from build123d import *

# Parameters (mm, degrees)
SKETCH_1_W          = 15.8
SKETCH_1_H          = 7.8
SKETCH_1_R          = 2.4
EXTRUDE_1_DEPTH     = 3.2
SKETCH_2_R          = 2.4
SKETCH_2_R_2        = 1.6
EXTRUDE_2_DEPTH     = 1.7
SKETCH_3_R          = 2.5
CUT_EXTRUDE_2_DEPTH = 1.8


with BuildPart() as part:
    # Эскиз1 → Бобышка-Вытянуть1 (new body)
    # profile 1 of 2: a face of its own
    with BuildSketch(Plane(origin=(0, 0, 0), x_dir=(1, 0, 0), z_dir=(0, 1, 0))):
        Rectangle(SKETCH_1_W, SKETCH_1_H)
        Circle(SKETCH_1_R, mode=Mode.SUBTRACT)
    # profile 2 of 2: a face of its own
    with BuildSketch(Plane(origin=(0, 0, 0), x_dir=(1, 0, 0), z_dir=(0, 1, 0))):
        Circle(SKETCH_1_R)
    extrude(amount=EXTRUDE_1_DEPTH)

    # Эскиз2 → Бобышка-Вытянуть2 (add)
    with BuildSketch(Plane(origin=(0, 0, 0), x_dir=(1, 0, 0), z_dir=(0, 1, 0))):
        with Locations(Location((0, 0, 0), (0, 0, 270))):
            Circle(SKETCH_2_R)
        with Locations(Location((0, 0, 0), (0, 0, 270))):
            Circle(SKETCH_2_R_2, mode=Mode.SUBTRACT)
    extrude(amount=-EXTRUDE_2_DEPTH)

    # Эскиз3 → Вырез-Вытянуть2 (cut)
    with BuildSketch(Plane(origin=(0, 3.2, 0), x_dir=(1, 0, 0), z_dir=(0, 1, 0))):
        with Locations(Location((-4, 0, 0), (0, 0, 270))):
            Circle(SKETCH_3_R)
        with Locations(Location((4, 0, 0), (0, 0, 270))):
            Circle(SKETCH_3_R)
    extrude(amount=-CUT_EXTRUDE_2_DEPTH, mode=Mode.SUBTRACT)


solid = part.part
The model under review builds one solid part; all positions refer to its coordinate system, in mm. A direction names the side the tool comes from. Round coordinates to 2 decimals unless told otherwise and drop trailing zeros. Order: outer loops, then holes, each group sorted by start corner. A loop starts at its lowest first (then second) coordinate and runs counter-clockwise, first axis right, second up. Notation, with made-up numbers: (-32, 41.25) -> (5, 41.25) arc R15 cw to (5, 62.25) -> close; hole circle Ø1 at (-21, 46). An arc over 180 degrees is marked (long way). Return JSON: item names as keys, results as strings.
1. For L1, parallel to X at y = 2.7, z = 0; L2, parallel to X at y = -0.35, z = 0; L3, parallel to X at y = 2.4, z = -0.75, list the stretches that pass through material, from the lowest coordinate up. Write a range as [from, to].
Answer block:
{"L1": "x = [-7.9, -6.5], [-1.5, 1.5], [6.5, 7.9]", "L2": "x = [-2.4, -1.6], [1.6, 2.4]", "L3": "x = [-7.9, -6.38], [-1.62, 1.62], [6.38, 7.9]"}
2. Take a section at C-C (y = 2.85). Write out the cut boundary in (x, z).
Answer block:
{"outline": "(-7.9, -3.9) -> (7.9, -3.9) -> (7.9, 3.9) -> (-7.9, 3.9) -> close; hole circle Ø5 at (-4, 0); hole circle Ø5 at (4, 0)"}
3. Take a section at A-A (z = 0). Write out the cut boundary in (x, y), then the cut area to 3 significant figures.
Answer block:
{"outline": "(-7.9, 0) -> (-2.4, 0) -> (-2.4, -1.7) -> (-1.6, -1.7) -> (-1.6, 0) -> (1.6, 0) -> (1.6, -1.7) -> (2.4, -1.7) -> (2.4, 0) -> (7.9, 0) -> (7.9, 3.2) -> (6.5, 3.2) -> (6.5, 1.4) -> (1.5, 1.4) -> (1.5, 3.2) -> (-1.5, 3.2) -> (-1.5, 1.4) -> (-6.5, 1.4) -> (-6.5, 3.2) -> (-7.9, 3.2) -> close", "area": "35.3 mm²"}
4. Take a section at D-D (y = -1.2). Write out the cut boundary in (x, z).
Answer block:
{"outline": "circle Ø4.8 at (0, 0); hole circle Ø3.2 at (0, 0)"}
5. For faces 4 (the face through (0, 0, 0)), 5 (the face through (0, 2, -3.9)), 6 (the face through (4, 1.4, 0)), list the 3-axis set-ups (+Z, -Z, +X, -X, +Y, -Y) from which the entire face can be reached by the end or side of a thin tool; tool diameter is ignored.
Answer block:
{"face 4": "-Y", "face 5": "-Z, +X, -X, +Y, -Y", "face 6": "+Y"}
6. The part is to be moulded in two halves that separate along X. For faces 1 (the face through (-2, -1.7, 0)), 2 (the face through (7.9, 2, 0)), 3 (the face through (-1.52, 2.31, -0.33)), say which applies: +X half, -X half, draft (parallel to the pull), parting line (faces both ways), or undercut.
Answer block:
{"face 1": "draft", "face 2": "+X half", "face 3": "undercut"}
7. Take a section at B-B (x = 4). Write out the cut boundary in (y, z).
Answer block:
{"outline": "(0, -3.9) -> (3.2, -3.9) -> (3.2, -2.5) -> (1.4, -2.5) -> (1.4, 2.5) -> (3.2, 2.5) -> (3.2, 3.9) -> (0, 3.9) -> close"}
8. Insertion check: P1, Ø1.5, axis at x = -3, z = -1, coming from the +Y side; P2, Ø2.5, axis at x = -1, z = 0, coming from the -Y side; P3, Ø2.5, axis at x = 0, z = 0, coming from the -Y side. Each pin has a flat end and moves straight along its axis. Give the tip position at first contact, or say it passes through.
Answer block:
{"P1": "stops at y = 1.4", "P2": "stops at y = -1.7", "P3": "stops at y = 0"}
